```python
from build123d import *

# Parameters (mm, degrees)
SKETCH_1_W      = 49.5
SKETCH_1_H      = 85
EXTRUDE_1_DEPTH = 5
SKETCH_12_W     = 15
SKETCH_12_H     = 5
EXTRUDE_3_DEPTH = 5


with BuildPart() as part:
    # 스케치1 → 보스-돌출1 (new body)
    with BuildSketch(Plane(origin=(0, 0, 0), x_dir=(0, 0, -1), z_dir=(1, 0, 0))):
        with Locations((24.75, 0.767010447)):
            Rectangle(SKETCH_1_W, SKETCH_1_H)
    extrude(amount=EXTRUDE_1_DEPTH)

    # 스케치12 → 보스-돌출3 (add)
    with BuildSketch(Plane(origin=(5, 0, 0), x_dir=(0, 0, -1), z_dir=(1, 0, 0))):
        with Locations((42, -44.232989553)):
            Rectangle(SKETCH_12_W, SKETCH_12_H)
        with Locations((7.5, -44.232989553)):
            Rectangle(SKETCH_12_W, SKETCH_12_H)
    extrude(amount=-EXTRUDE_3_DEPTH)


solid = part.part
```
Model file for the job. Use its own axes, mm. A direction names the side the tool comes from. Coordinates: 2 decimals unless noted, no trailing zeros. Order: outer loops, then holes, each group sorted by start corner. A loop starts at its lowest first (then second) coordinate and runs counter-clockwise, first axis right, second up. Notation, with made-up numbers: (5.25, -37) -> (27.25, -37) arc R24 ccw to (27.25, 2) -> close; hole circle Ø9 at (6.5, 87). An arc over 180 degrees is marked (long way). Answer as a JSON object with one key per item and string values. Group by question number.
1) Drill centre line: L1, parallel to Y at x = 3.65, z = -28. Where is it in solid material? Low to high.
2) Cut at B-B, the plane z = -31.5. Write the cut outline in (x, y), then the cut area to 3 significant figures.
3) Flat gauge pin, fed straight in: pin 1 (8 mm diameter, centred on y = -5, z = -13.5, fed in from -X). Where does the tip first touch, or does it go through?
4) Cut at A-A, the plane x = 1.1. Write the cut outline in (y, z), then the cut area to 3 significant figures.
5) Pull direction Z, two halves, no side cores. Call faces 3 (the face through (3, -46.733, -42)), 4 (the face through (3, -44, -34.5)), 5 (the face through (2, -2, 0)): +Z half, -Z half, draft (parallel to the pull), parting line (faces both ways), or undercut.
6) Which spindle directions (+Z, -Z, +X, -X, +Y, -Y) get a long thin tool onto all of the face, cutting with end or side? Do faces 1 (the face through (2, 43.267, -24)), 2 (the face through (3, -44, -15)). Say none if no direction does.
Check values:
{
 "1": {"L1": "y = -41.73 to 43.27"},
 "2": {"outline": "(0, -41.73) -> (5, -41.73) -> (5, 43.27) -> (0, 43.27) -> close", "area": "425 mm²"},
 "3": {"pin 1": "stops at x = 0"},
 "4": {"outline": "(-46.73, -49.5) -> (43.27, -49.5) -> (43.27, 0) -> (-46.73, 0) -> (-46.73, -15) -> (-41.73, -15) -> (-41.73, -34.5) -> (-46.73, -34.5) -> close", "area": "4,360 mm²"},
 "5": {"face 3": "draft", "face 4": "undercut", "face 5": "+Z half"},
 "6": {"face 1": "+Z, -Z, +X, -X, +Y", "face 2": "+X, -X, -Y"}
}
